Design review of the part built by this model. Coordinates are the model's own, in mm. A direction names the side the tool comes from. Round coordinates to 2 decimals unless told otherwise and drop trailing zeros. Loops run counter-clockwise (first coordinate to the right, second up) from the corner with the lowest first, then second, coordinate; pieces in that order, holes last. Notation, with made-up numbers: M 36,64 L 76,64 A16 ccw 76,92 Z; hole C 49,-34.5 d4. An arc over 180 degrees is marked long. One line per item, written item: value. Start each with the question number.
Item 1: Mouldability with a two-part tool opening along Z and no side actions: class faces 3 (the cylindrical face through (37.92, -0.69, -15.74)), 4 (the cylindrical face through (25.756, 6.456, -1.434)), 5 (the cylindrical face through (42.965, 10.98, 0.572)), 6 (the flat face through (25.4, 11, 12)) as released by +Z, released by -Z, zero draft, split by the parting line, or undercut.
Item 2: We need section C-C (x = 8.5). Write out the cut boundary in (y, z), then the cut area to 3 significant figures.
Item 3: Clearance check with flat-ended pins moving along their axes: pin 1 (5 mm diameter, centred on x = 41.148, z = 0, fed in from +Y); pin 2 (5 mm diameter, centred on x = 28, y = 1, fed in from +Z); pin 3 (5 mm diameter, centred on y = -27.5, z = -12, fed in from -X); pin 4 (1 mm diameter, centred on y = 3, z = 33.5, fed in from +X). State where each tip first meets the part, or that it passes through.
Item 4: We need section D-D (x = 38). Write out the cut boundary in (y, z).
Item 5: We need section B-B (y = 0). Write out the cut boundary in (x, z), then the cut area to 3 significant figures.
Item 6: For line 1 along Y through (x, z) = (11, 0); line 2 along X through (y, z) = (13, 0), list the stretches that pass through material, from the lowest coordinate up.
Item 7: We need section A-A (z = 0). Write out the cut boundary in (x, y).
Item 8: For faces 1 (the conical face through (5.036, -13.405, 42.566)), 2 (the flat face through (50.8, 7, 0)), list the 3-axis set-ups (+Z, -Z, +X, -X, +Y, -Y) from which the entire face can be reached by the end or side of a thin tool; tool diameter is ignored.
from build123d import *

# Parameters (mm, degrees)
F2_R     = 1.905
F3_DEPTH = 25.4


with BuildPart() as f1:
    # F0 (on Front) → F1 (revolve)
    with BuildSketch(Plane.XZ):
        Polygon((0, 50.761004), (0, 6.612969), (50.8, 6.612969), (50.8, 15.756969), (25.4, 15.756969), (25.4, 50.808969), (22.098, 50.808969), (20.42762, 44.217008), (5.151389, 44.217008), (3.302, 50.761004), align=None)
    revolve(axis=Axis((50.224784, 0, 0), (1, 0, 0)))

    # F2 (on Front) → F3 (cut)
    with BuildSketch(Plane.XZ):
        with Locations((41.148, 0)):
            Circle(F2_R)
    extrude(amount=-F3_DEPTH, mode=Mode.SUBTRACT)


solid = f1.part
A:
1. face 3: split by the parting line
1. face 4: undercut
1. face 5: undercut
1. face 6: zero draft
2. outline: C 0,0 d88.43; hole C 0,0 d13.23
2. area: 6,000 mm2
3. pin 1: y = 15.76
3. pin 2: z = 15.76
3. pin 3: x = 0
3. pin 4: x = 25.4
4. outline: C 0,0 d31.51; hole C 0,0 d13.23
5. outline: M 0,-50.76 L 3.3,-50.76 L 5.15,-44.22 L 20.43,-44.22 L 22.1,-50.81 L 25.4,-50.81 L 25.4,-15.76 L 50.8,-15.76 L 50.8,-6.61 L 0,-6.61 Z; M 0,6.61 L 50.8,6.61 L 50.8,15.76 L 25.4,15.76 L 25.4,50.81 L 22.1,50.81 L 20.43,44.22 L 5.15,44.22 L 3.3,50.76 L 0,50.76 Z
5. area: 2,480 mm2
6. line 1: -44.22 to -6.61, 6.61 to 44.22
6. line 2: 0 to 39.24, 43.05 to 50.8
7. outline: M 0,-50.76 L 3.3,-50.76 L 5.15,-44.22 L 20.43,-44.22 L 22.1,-50.81 L 25.4,-50.81 L 25.4,-15.76 L 50.8,-15.76 L 50.8,-6.61 L 0,-6.61 Z; M 0,6.61 L 39.24,6.61 L 39.24,15.76 L 25.4,15.76 L 25.4,50.81 L 22.1,50.81 L 20.43,44.22 L 5.15,44.22 L 3.3,50.76 L 0,50.76 Z; M 43.05,6.61 L 50.8,6.61 L 50.8,15.76 L 43.05,15.76 Z
8. face 1: none
8. face 2: +Z, -Z, +X, +Y, -Y
